```python
from build123d import *

# Parameters (mm, degrees)
SZKIC1_R                    = 10
DODANIE_WYCI_GNI_CIE1_DEPTH = 900
SZKIC2_R                    = 10
SZKIC2_R_2                  = 7.5
WYTNIJ_WYCI_GNI_CIE1_DEPTH  = 65
SZKIC3_R                    = 10
SZKIC3_R_2                  = 6
WYTNIJ_WYCI_GNI_CIE2_DEPTH  = 18
SFAZOWANIE1_SIZE            = 0.5
SFAZOWANIE2_SIZE            = 0.3
SFAZOWANIE3_SIZE            = 0.5
WYTNIJ_WYCI_GNI_CIE3_DEPTH  = 20


with BuildPart() as part:
    # Szkic1 → Dodanie-wyciągnięcie1 (new body)
    with BuildSketch(Plane.XY):
        Circle(SZKIC1_R)
    extrude(amount=DODANIE_WYCI_GNI_CIE1_DEPTH)

    # Szkic2 → Wytnij-wyciągnięcie1 (cut)
    with BuildSketch(Plane.XY.offset(900)):
        Circle(SZKIC2_R)
        Circle(SZKIC2_R_2, mode=Mode.SUBTRACT)
    extrude(amount=-WYTNIJ_WYCI_GNI_CIE1_DEPTH, mode=Mode.SUBTRACT)

    # Szkic3 → Wytnij-wyciągnięcie2 (cut)
    with BuildSketch(Plane.XY.offset(900)):
        Circle(SZKIC3_R)
        Circle(SZKIC3_R_2, mode=Mode.SUBTRACT)
    extrude(amount=-WYTNIJ_WYCI_GNI_CIE2_DEPTH, mode=Mode.SUBTRACT)

    # Sfazowanie1
    sfazowanie1_edges = [part.edges().sort_by_distance(p)[0] for p in [
        (-10, 0, 835),
    ]]
    chamfer(sfazowanie1_edges, length=SFAZOWANIE1_SIZE)

    # Sfazowanie2
    sfazowanie2_edges = [part.edges().sort_by_distance(p)[0] for p in [
        (-7.5, 0, 882),
        (-6, 0, 900),
    ]]
    chamfer(sfazowanie2_edges, length=SFAZOWANIE2_SIZE)

    # Sfazowanie3
    sfazowanie3_edges = [part.edges().sort_by_distance(p)[0] for p in [
        (-10, 0, 0),
    ]]
    chamfer(sfazowanie3_edges, length=SFAZOWANIE3_SIZE)

    # Szkic4 → Wytnij-wyciągnięcie3 (cut)
    with BuildSketch(Plane.XY.offset(882)):
        Polygon((0, 6), (2, 6), (2, 8.058022447), (-2, 8.058022447), (-2, 6), align=None)
    extrude(amount=-WYTNIJ_WYCI_GNI_CIE3_DEPTH, mode=Mode.SUBTRACT)


solid = part.part
```
Source: CAD feature listing. Evaluate the final solid. Frame: model axes, mm. A direction names the side the tool comes from. Give positions to 0.01 mm unless a question says otherwise; leave off trailing zeros. Order: outer loops, then holes, each group sorted by start corner. A loop starts at its lowest first (then second) coordinate and runs counter-clockwise, first axis right, second up. Notation, with made-up numbers: (-37.5, 28.25) -> (10.5, 28.25) arc R27 cw to (10.5, 44.25) -> close; hole circle Ø9 at (-21, 69.25). An arc over 180 degrees is marked (long way). Use a Markdown table: item, result.
Q1. Section B-B (z = 467). Return the cut outline in (x, y), and give its area (3 significant figures).
A:
| item | result |
|---|---|
| outline | circle Ø20 at (0, 0) |
| area | 314 mm^2 |
Q2. Section A-A (y = 0). Return the cut outline in (x, z), and give its area (3 significant figures).
A:
| item | result |
|---|---|
| outline | (-10, 0.5) -> (-9.5, 0) -> (9.5, 0) -> (10, 0.5) -> (10, 834.5) -> (9.5, 835) -> (7.5, 835) -> (7.5, 881.7) -> (7.2, 882) -> (6, 882) -> (6, 899.7) -> (5.7, 900) -> (-5.7, 900) -> (-6, 899.7) -> (-6, 882) -> (-7.2, 882) -> (-7.5, 881.7) -> (-7.5, 835) -> (-9.5, 835) -> (-10, 834.5) -> close |
| area | 17,600 mm^2 |
Q3. Access query for faces 1 (the face through (-2.17, -9.76, 411.66)), 2 (the face through (2, -6, 882)). Directions: +Z, -Z, +X, -X, +Y, -Y. A direction counts if a zero-diameter tool reaches every point of the face in a straight line with its end or side. Return the directions, or none.
A:
| item | result |
|---|---|
| face 1 | +Z, -Z |
| face 2 | +Z |
Q4. Material intervals for line 1 (X direction, y = 1.75, z = 530); line 2 (Z direction, x = -8.75, y = -0.25); line 3 (X direction, y = 6.75, z = 62), sorted ascending. Write a range as [from, to].
A:
| item | result |
|---|---|
| line 1 | [-9.85, 9.85] |
| line 2 | [0, 835] |
| line 3 | [-7.38, 7.38] |
Q5. First-contact query: P1, Ø8, axis at x = -6, z = 580.5, coming from the +Y side; P2, Ø1.4, axis at y = 6.5, z = 873, coming from the -X side (3 decimals); P3, Ø1.2, axis at x = 0.5, y = 7, coming from the +Z side. Flat tips, straight axial feed; report the tip coordinate or a pass-through.
A:
| item | result |
|---|---|
| P1 | y = 9.8 |
| P2 | x = -4.755 |
| P3 | z = 862 |
